```python
from build123d import *

# Parameters (mm, degrees)
F1_DEPTH      = 55
F1_DEPTH_BACK = 55
F4_DEPTH      = 3
F6_W          = 90
F6_H          = 116
F7_DEPTH      = 3
F9_W          = 116
F9_H          = 13
F10_DEPTH     = 3
F13_DEPTH     = 10


# Not quite as in the source:
# - a pattern or mirror of a feature is missing from the dataset's text; its kind, count and spacing are read off the source's solid


with BuildPart() as f1:
    # F0 (on Front) → F1 (new body, two sides)
    with BuildSketch(Plane.XZ) as f1_sk:
        Polygon((-49.7641339898, 203), (-49.7641339898, 0), (243.2358660102, 0), (243.2358660102, 3), (-46.7641339898, 3), (-46.7641339898, 203), align=None)
    extrude(amount=F1_DEPTH)
    extrude(f1_sk.sketch, amount=-F1_DEPTH_BACK)

    # F3 (on offset) → F4 (join)
    with BuildSketch(Plane.XZ.offset(55)):
        Polygon((40.2358660102, 203), (-49.7641339898, 203), (-49.7641339898, 0), (243.2358660102, 0), (243.2358660102, 13), (40.2358660102, 13), align=None)
    f4 = extrude(amount=F4_DEPTH)

    # F4_copies: F4 across plane
    add(f4.mirror(Plane.ZX))

    # F6 (on face) → F7 (join)
    with BuildSketch(Plane.XY.offset(203)):
        with Locations((-4.7641339898, 0)):
            Rectangle(F6_W, F6_H)
    extrude(amount=F7_DEPTH)

    # F9 (on face) → F10 (join)
    with BuildSketch(Plane.YZ.offset(243.2358660102)):
        with Locations((0, 6.5)):
            Rectangle(F9_W, F9_H)
    extrude(amount=F10_DEPTH)

    # F12 (on offset) → F13 (join)
    with BuildSketch(Plane.XY.offset(3)):
        with BuildLine():
            Line((210.3120674863, 29.9101863056), (210.3120674863, 0))
            Line((210.3120674863, 0), (210.3120674863, -29.9101863056))
            ThreePointArc((210.3120674863, -29.9101863056), (216.7739667483, -36.3720855676), (223.2358660102, -29.9101863056))
            Line((223.2358660102, -29.9101863056), (223.2358660102, 0))
            Line((223.2358660102, 0), (223.2358660102, 29.9101863056))
            ThreePointArc((223.2358660102, 29.9101863056), (216.7739667483, 36.3720855676), (210.3120674863, 29.9101863056))
        make_face()
    extrude(amount=F13_DEPTH)


solid = f1.part
```
Verification items for the finished model (mm, model axes). A direction names the side the tool comes from. Coordinates: 2 decimals unless noted, no trailing zeros. Order: outer loops, then holes, each group sorted by start corner. A loop starts at its lowest first (then second) coordinate and runs counter-clockwise, first axis right, second up. Notation, with made-up numbers: (64, -20) - (120, -20) arc R15 cw to (120, 4) - close; hole circle Ø2 at (-20.5, 50.5). An arc over 180 degrees is marked (long way). Return JSON: item names as keys, results as strings.
(1) Section check D-D, the plane x = 52. Record the cut outline in (y, z), and give its area (3 significant figures).
Filled sheet:
{"outline": "(-58, 0) - (58, 0) - (58, 13) - (55, 13) - (55, 3) - (-55, 3) - (-55, 13) - (-58, 13) - close", "area": "408 mm^2"}
(2) Thickness scan on line 1 along Y through (x, z) = (20, 146); line 2 along Z through (x, y) = (9.5, -3); line 3 along X through (y, z) = (39, 12). Record the ranges inside material, lowest first.
Filled sheet:
{"line 1": "y = -58 to -55, 55 to 58", "line 2": "z = 0 to 3, 203 to 206", "line 3": "x = -49.76 to -46.76, 243.24 to 246.24"}
(3) Section check A-A, the plane x = 19.5. Record the cut outline in (y, z), and give its area (3 significant figures).
Filled sheet:
{"outline": "(-58, 0) - (58, 0) - (58, 206) - (-58, 206) - close; hole (-55, 3) - (55, 3) - (55, 203) - (-55, 203) - close", "area": "1,900 mm^2"}
(4) Section check B-B, the plane y = -20.5. Record the cut outline in (x, z), and give its area (3 significant figures).
Filled sheet:
{"outline": "(-49.76, 0) - (246.24, 0) - (246.24, 13) - (243.24, 13) - (243.24, 3) - (223.24, 3) - (223.24, 13) - (210.31, 13) - (210.31, 3) - (-46.76, 3) - (-46.76, 203) - (40.24, 203) - (40.24, 206) - (-49.76, 206) - close", "area": "1,920 mm^2"}
(5) Access from +Z, -Z, +X, -X, +Y, -Y to the whole of each face (thin tool, end or side, straight path). Record for faces 1 (the flat face through (100, -1, 3)), 2 (the flat face through (-5, 1, 206)), 3 (the flat face through (217, 1, 13)), 4 (the flat face through (-49.764, -1, 102)), 5 (the flat face through (210.312, 0, 8)).
Filled sheet:
{"face 1": "none", "face 2": "+Z, +X, -X, +Y, -Y", "face 3": "+Z, +X, +Y, -Y", "face 4": "+Z, -Z, -X, +Y, -Y", "face 5": "+Z"}
(6) Go/stop test with flat-tipped pins: pin 1 (1 mm diameter, centred on x = 146.5, y = 26.5, fed in from +Z); pin 2 (10 mm diameter, centred on y = -5, z = 123, fed in from +X); pin 3 (4 mm diameter, centred on x = 215.5, y = 8.5, fed in from +Z). Record where each tip stops, or that it passes through.
Filled sheet:
{"pin 1": "stops at z = 3", "pin 2": "stops at x = -46.76", "pin 3": "stops at z = 13"}
(7) Section check C-C, the plane z = 183. Record the cut outline in (x, y), and give its area (3 significant figures).
Filled sheet:
{"outline": "(-49.76, -58) - (40.24, -58) - (40.24, -55) - (-46.76, -55) - (-46.76, 55) - (40.24, 55) - (40.24, 58) - (-49.76, 58) - close", "area": "870 mm^2"}
(8) Mould release check, pull along Z, two halves, no side actions. Record for faces 6 (the flat face through (96, -1, 0)), 7 (the flat face through (12, -55, 96)), 8 (the flat face through (243.236, -1, 8)), 9 (the flat face through (-4, 1, 203)): pulls with the +Z half, pulls with the -Z half, needs draft (parallel to the pull), parting line crosses it, or undercut.
Filled sheet:
{"face 6": "pulls with the -Z half", "face 7": "undercut", "face 8": "needs draft", "face 9": "undercut"}
